CAD build for the part. Positions are in the model's coordinates, mm. Face numbers are marked on the shaded views. A direction names the side the tool comes from. Give positions to 0.01 mm unless a question says otherwise; leave off trailing zeros. Write each loop counter-clockwise with the first axis right and the second up, starting at its lowest first coordinate (ties: lowest second). Pieces come first, ordered by that corner, then holes. Notation, with made-up numbers: (66, 18) - (75, 18) arc R20 ccw to (75, 43) - close; hole circle Ø7 at (60.25, -32.5). An arc over 180 degrees is marked (long way). Write item = value, one per line. Start each with the question number.
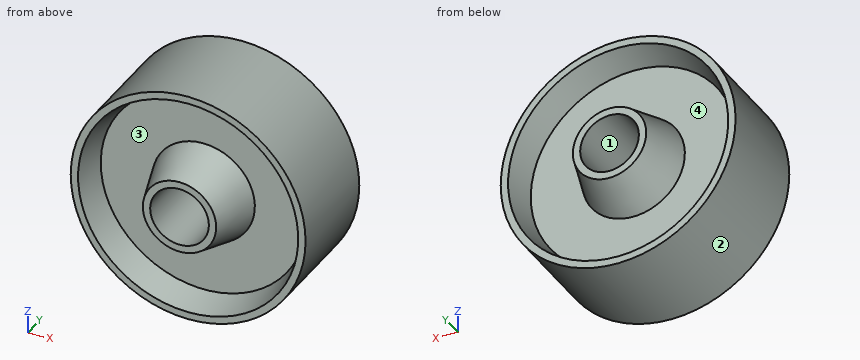
```python
from build123d import *


with BuildPart() as f1:
    # F0 (on Right) → F1 (revolve)
    with BuildSketch(Plane.YZ):
        Polygon((-46.801966, 39.576525), (-46.801966, 36.401525), (-26.958216, 36.401525), (-26.958216, 45.926525), align=None)
        Polygon((-26.958216, 45.926525), (-26.958216, 36.401525), (-7.908216, 36.401525), (-7.908216, 45.926525), (-7.908216, 68.151525), (-7.908216, 74.501525), (-17.433216, 74.501525), (-26.958216, 74.501525), (-26.958216, 68.151525), align=None)
        Polygon((-7.908216, 45.926525), (-7.908216, 36.401525), (11.935534, 36.401525), (11.935534, 39.576525), align=None)
        Polygon((-39.658216, 71.326525), (-26.958216, 68.151525), (-26.958216, 74.501525), (-39.658216, 74.501525), align=None)
        Polygon((-7.908216, 74.501525), (-7.908216, 68.151525), (4.791784, 71.326525), (4.791784, 74.501525), align=None)
    revolve(axis=Axis((0, 4.550466, 23.701525), (0, 1, 0)))


solid = f1.part
```
1. Cut at B-B (y = -3.5). Give the cut face in (x, z).
2. Cut at A-A (x = 0). Give the cut face in (y, z).
3. Cut at C-C (y = -14.5). Give the cut face in (x, z), then the cut area to 3 significant figures.
4. Pin check, flat tips, straight feed: pin 1 Ø1 at (x, y) = (-30.5, -23) entering from -Z; pin 2 Ø5 at (x, z) = (33, 16) entering from +Y; pin 3 Ø3 at (x, y) = (35, 1) entering from +Z; pin 4 Ø20.5 at (x, z) = (0, 23.7) entering from +Y (1 decimal). Stop position of each tip, or through.
5. Tool access for the marked faces 3 and 4: list every direction of +Z, -Z, +X, -X, +Y, -Y with a clear straight run to the whole face (end or side of a thin tool).
6. Wall check: line 1 along X through (y, z) = (-27, 41); line 2 along X through (y, z) = (-0.5, 23.5); line 3 along X through (y, z) = (-36, 21.5). Give the ranges that are in metal, low to high.
7. Mould opens along Z. For the marked faces 1 and 2 say: +Z half, -Z half, draft (parallel to the pull), parting line (faces both ways), or undercut.
Output:
q1.outline = circle Ø101.6 at (0, 23.7); circle Ø41.63 at (0, 23.7); hole circle Ø91.1 at (0, 23.7); hole circle Ø25.4 at (0, 23.7)
q2.outline = (-46.8, 7.83) - (-26.96, 1.48) - (-26.96, -20.75) - (-39.66, -23.92) - (-39.66, -27.1) - (4.79, -27.1) - (4.79, -23.92) - (-7.91, -20.75) - (-7.91, 1.48) - (11.94, 7.83) - (11.94, 11) - (-46.8, 11) - close; (-46.8, 36.4) - (11.94, 36.4) - (11.94, 39.58) - (-7.91, 45.93) - (-7.91, 68.15) - (4.79, 71.33) - (4.79, 74.5) - (-39.66, 74.5) - (-39.66, 71.33) - (-26.96, 68.15) - (-26.96, 45.93) - (-46.8, 39.58) - close
q3.outline = circle Ø101.6 at (0, 23.7); hole circle Ø25.4 at (0, 23.7)
q3.area = 7,600 mm2
q4.pin_1 = -17.29
q4.pin_2 = -7.91
q4.pin_3 = 61.89
q4.pin_4 = through
q5.face_3 = -Y
q5.face_4 = +Y
q6.line_1 = -47.76 to -40.96, -13.93 to 13.93, 40.96 to 47.76
q6.line_2 = -50.8 to -46.3, -19.85 to -12.7, 12.7 to 19.85, 46.3 to 50.8
q6.line_3 = -50.75 to -46.66, -19.21 to -12.51, 12.51 to 19.21, 46.66 to 50.75
q7.face_1 = undercut
q7.face_2 = parting line
